CAD build for the part. Positions are in the model's coordinates, mm. A direction names the side the tool comes from. Round coordinates to 2 decimals unless told otherwise and drop trailing zeros. Loops run counter-clockwise (first coordinate to the right, second up) from the corner with the lowest first, then second, coordinate; pieces in that order, holes last. Notation, with made-up numbers: (31.25, 34) - (36.25, 34) arc R21 cw to (36.25, 49) - close; hole circle Ø9 at (43, 44). An arc over 180 degrees is marked (long way). One line per question, with ' | ' between items.
Autodesk Inventor part; units mm, degrees
ref_plane "YZ Plane" through (0, 0, 0) normal (1, 0, 0) x (0, 1, 0)
ref_plane "XZ Plane" through (0, 0, 0) normal (0, 1, 0) x (-1, 0, 0)
ref_plane "XY Plane" through (0, 0, 0) normal (0, 0, 1) x (1, 0, 0)
sketch "Skizze1" plane through (0, 0, 0) normal (0, 1, 0) x (-1, 0, 0)
  line L0 (-101.4396, -103.5796) -> (-101.4396, -93.5796)
  line L1 (-101.4396, -93.5796) -> (48.5604, -93.5796)
  line L2 (48.5604, -93.5796) -> (48.5604, -103.5796)
  line L3 (-176.4396, -103.5796) -> (-101.4396, -103.5796)
  line L4 (48.5604, -103.5796) -> (123.5604, -103.5796)
  line L5 (-101.4396, 51.4204) -> (-101.4396, 41.4204)
  line L6 (-101.4396, 41.4204) -> (48.5604, 41.4204)
  line L7 (48.5604, 41.4204) -> (48.5604, 51.4204)
  line L8 (123.5604, 51.4204) -> (48.5604, 51.4204)
  line L9 (-101.4396, 51.4204) -> (-176.4396, 51.4204)
  line L10 (123.5604, 11.4204) -> (133.5604, 11.4204)
  line L11 (133.5604, 11.4204) -> (133.5604, -63.5796)
  line L12 (133.5604, -63.5796) -> (123.5604, -63.5796)
  line L13 (123.5604, -103.5796) -> (123.5604, -63.5796)
  line L14 (123.5604, 11.4204) -> (123.5604, 51.4204)
  line L15 (48.5604, -8.5796) -> (-101.4396, -8.5796)
  line L16 (-101.4396, -8.5796) -> (-101.4396, -18.5796)
  line L17 (-101.4396, -18.5796) -> (48.5604, -18.5796)
  line L18 (48.5604, -18.5796) -> (48.5604, -8.5796)
  line L19 (-176.4396, 11.4204) -> (-186.4396, 11.4204)
  line L20 (-186.4396, 11.4204) -> (-186.4396, -63.5796)
  line L21 (-186.4396, -63.5796) -> (-176.4396, -63.5796)
  line L22 (-176.4396, 51.4204) -> (-176.4396, 11.4204)
  line L23 (-176.4396, -63.5796) -> (-176.4396, -103.5796)
  dimension "d0" = 300
  dimension "d2" = 150
  dimension "d3" = 10
  dimension "d6" = 10
  dimension "d7" = 10
  dimension "d8" = 75
  dimension "d10" = 150
  dimension "d11" = 10
  dimension "d13" = 10
  dimension "d14" = 75
  dimension "d17" = 10
  dimension "d20" = 10
  dimension "d22" = 50
  dimension "d25" = 155
  dimension "d26" = 0
  dimension "d27" = 10
  dimension "d28" = 40
  dimension "d29" = 40
  dimension "d30" = 85
  dimension "d31" = 75
  dimension "d32" = 85
  dimension "d33" = 75
  dimension "d34" = 10
  dimension "d35" = 150
extrude "Extrusion1" add sketch "Skizze1" along normal blind 10
properties part number "Platte3-Seite"
(1) Cut at C-C, the plane z = -15. Write the cut outline in (x, y), then the cut area to 3 significant figures.
Results found:
outline: (-133.56, 0) - (-48.56, 0) - (-48.56, 10) - (-133.56, 10) - close; (101.44, 0) - (186.44, 0) - (186.44, 10) - (101.44, 10) - close | area: 1,700 mm²
(2) Probe L1, parallel to Z at x = 2, y = 3.5; L2, parallel to X at y = 1.5, z = -18.5; L3, parallel to X at y = 3.5, z = 42. List the from-to ranges inside material, lowest first.
Results found:
L1: z = -93.58 to -18.58, -8.58 to 41.42 | L2: x = -133.56 to -48.56, 101.44 to 186.44 | L3: x = -123.56 to -48.56, 101.44 to 176.44
(3) Drop flat-ended pins along their axis: P1, Ø5, axis at x = 11.5, y = 6, coming from the +Z side; P2, Ø4, axis at x = 20, y = 9, coming from the -Z side; P3, Ø3, axis at x = -16, z = -16, coming from the +Y side; P4, Ø3, axis at y = 7, z = 21.5, coming from the -X side. Give the stop position or say it passes through.
Results found:
P1: stops at z = 41.42 | P2: stops at z = -93.58 | P3: passes through | P4: stops at x = -123.56
(4) Cut at D-D, the plane z = 20. Write the cut outline in (x, y), then the cut area to 3 significant figures.
Results found:
outline: (-123.56, 0) - (176.44, 0) - (176.44, 10) - (-123.56, 10) - close | area: 3,000 mm²
(5) Cut at A-A, the plane y = 8.25. Write the cut outline in (x, z).
Results found:
outline: (-133.56, -63.58) - (-123.56, -63.58) - (-123.56, -103.58) - (-48.56, -103.58) - (-48.56, -93.58) - (101.44, -93.58) - (101.44, -103.58) - (176.44, -103.58) - (176.44, -63.58) - (186.44, -63.58) - (186.44, 11.42) - (176.44, 11.42) - (176.44, 51.42) - (101.44, 51.42) - (101.44, 41.42) - (-48.56, 41.42) - (-48.56, 51.42) - (-123.56, 51.42) - (-123.56, 11.42) - (-133.56, 11.42) - close; hole (-48.56, -18.58) - (101.44, -18.58) - (101.44, -8.58) - (-48.56, -8.58) - close
(6) Tool access for faces 1 (the face through (181, 5, 11.42)), 2 (the face through (101.44, 5, -99)), 3 (the face through (-123.56, 5, 31)), 4 (the face through (25, 5, -8.58)): list every direction of +Z, -Z, +X, -X, +Y, -Y with a clear straight run to the whole face (end or side of a thin tool).
Results found:
face 1: +Z, +X, +Y, -Y | face 2: -Z, +Y, -Y | face 3: +Z, -X, +Y, -Y | face 4: +Y, -Y
(7) Cut at B-B, the plane x = -3.5. Write the cut outline in (y, z), then the cut area to 3 significant figures.
Results found:
outline: (0, -93.58) - (10, -93.58) - (10, -18.58) - (0, -18.58) - close; (0, -8.58) - (10, -8.58) - (10, 41.42) - (0, 41.42) - close | area: 1,250 mm²
(8) Two-plate mould, pull along X, no slides. Class faces 5 (the face through (27, 5, 41.42)), 6 (the face through (176.44, 5, 32)), 7 (the face through (138, 5, 51.42)): released by +X, released by -X, zero draft, split by the parting line, or undercut.
Results found:
face 5: undercut | face 6: released by +X | face 7: zero draft
